The drawing under review shows one solid part. Ordinate dimensions are in mm from its lowest x, y, z. Coordinates: 2 decimals unless noted, no trailing zeros. Order: outer loops, then holes, each group sorted by start corner. A loop starts at its lowest first (then second) coordinate and runs counter-clockwise, first axis right, second up.
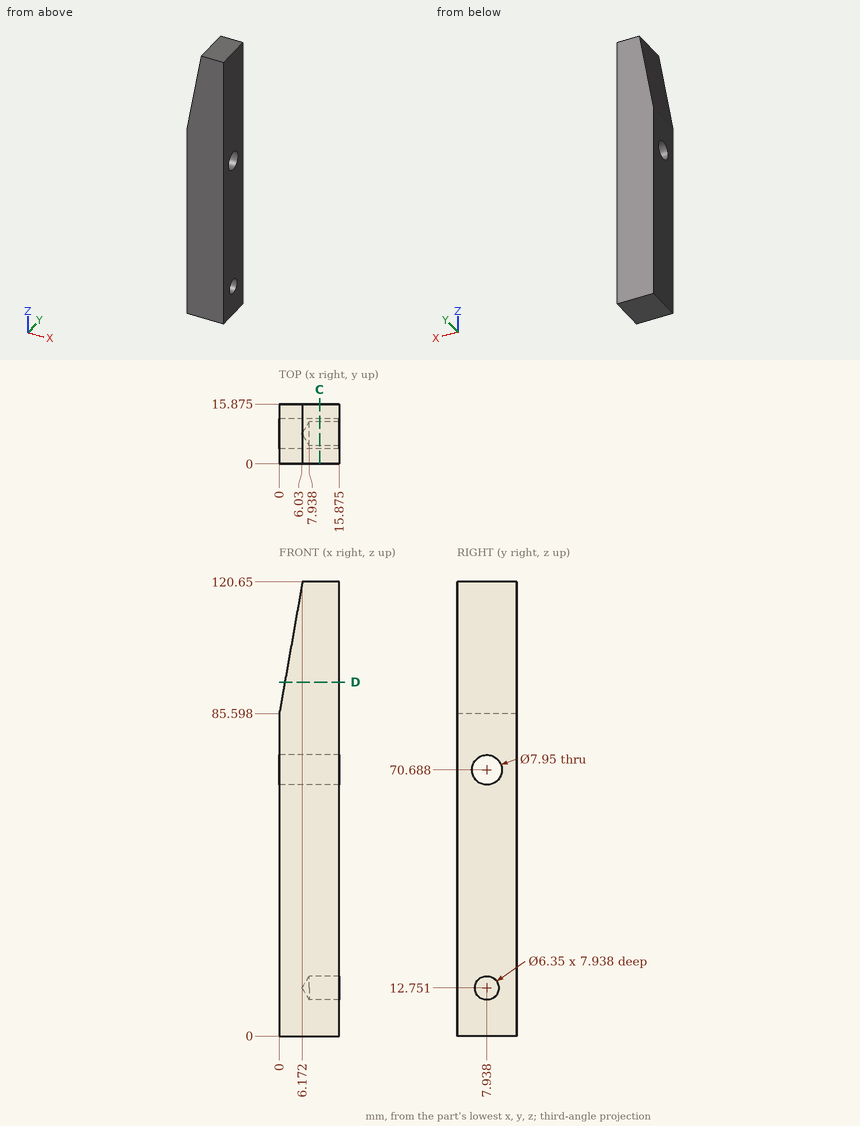
(1) We need section D-D, the plane z = 94. Write out the cut boundary in (x, y) (1 decimal).
A:
outline: (1.5, 0) - (15.9, 0) - (15.9, 15.9) - (1.5, 15.9) - close
(2) We need section C-C, the plane x = 10.75. Count the separate pieces of the cut face and the enclosed holes in it, and give its area (3 significant figures).
A:
separate pieces: 1
enclosed holes: 2
area: 1,830 mm2
(3) For pin 1 Ø2 at (y, z) = (12, 89) entering from -X, flat-tipped, find the tip position at first contact; note if it passes through.
A:
pin 1: stops at x = 0.42
(4) Wall thickness on probe 1 along Y at (x, z) = (3.25, 70.5) (1 decimal); probe 2 along Y at (x, z) = (5, 72) (1 decimal); probe 3 along X at (y, z) = (1.5, 101) (1 decimal): over which ranges is each line inside the solid? List them lowest first.
A:
probe 1: y = 0 to 4, 11.9 to 15.9
probe 2: y = 0 to 4.2, 11.7 to 15.9
probe 3: x = 2.7 to 15.9
